Can you work these out from the model? Positions are in its coordinate system, mm. A direction names the side the tool comes from. Coordinates: 2 decimals unless noted, no trailing zeros. Order: outer loops, then holes, each group sorted by start corner. A loop starts at its lowest first (then second) coordinate and runs counter-clockwise, first axis right, second up. Notation, with made-up numbers: (-13, 3.5) - (20, 3.5) arc R17 ccw to (20, 16.5) - close; hole circle Ø10 at (7, 7). An arc over 180 degrees is marked (long way). Use a Markdown table: item, result. Add a question column.
(1) I want a section at C-C (x = -7.5). List the corners of the cut face in (y, z) for me.
(2) We'd pull the mould along Z, two halves only. Please class faces 1 (the cylindrical face through (-35.639, -56.36, -108.857)), 2 (the cylindrical face through (-35.639, -56.36, -32.408)), 3 (the flat face through (0, -24, -10)), 4 (the cylindrical face through (23.66, -15.06, -4.93)): pulls with the +Z half, pulls with the -Z half, needs draft (parallel to the pull), parting line crosses it, or undercut.
(3) I want a section at A-A (z = -64.5). List the corners of the cut face in (x, y) for me, and give its area (3 significant figures).
(4) For pin 1 Ø8 at (y, z) = (-20.5, -3.5) entering from -X; pin 2 Ø11 at (y, z) = (-24.5, -3) entering from +X; pin 3 Ø1 at (x, z) = (0.5, -24.5) entering from +Y, each with a flat end and sliding along its axis, tell me the tip position at first contact or that it passes through.
(5) On a 3-axis mill with a long thin cutter (end or side, diameter ignored), from which of +Z, -Z, +X, -X, +Y, -Y can I reach the whole of each face in a straight line? I mean faces 5 (the flat face through (28.5, -23, -5)), 6 (the flat face through (-17.5, -37, -61)), 7 (the flat face through (17.5, -37, -61)), 8 (the flat face through (-28.5, 23, -5)). Say none if no direction works.
(6) I want a section at D-D (y = -31). List the corners of the cut face in (x, z) for me, and give its area (3 significant figures).
(7) If I drill on L1, parallel to Z at x = -34.5, y = -57; L2, parallel to Y at x = 12.5, z = -80.5; L3, parallel to Z at x = 22, y = 2, over which ranges is the centre line in solid material (lowest first)? Write a range as [from, to].
(8) I want a section at B-B (y = 15). List the corners of the cut face in (x, z) for me, and give its area (3 significant figures).
```python
from build123d import *

# Parameters (mm, degrees)
SKETCH3_W           = 57
SKETCH3_H           = 57
BOSS_EXTRUDE1_DEPTH = 10
SKETCH3_3_R         = 2.55
CUT_EXTRUDE1_DEPTH  = 10
BOSS_EXTRUDE2_DEPTH = 112
SKETCH4_R           = 19.05
SKETCH4_R_2         = 6.5
CUT_EXTRUDE2_DEPTH  = 129.967050055
SKETCH5_R           = 4.15
CUT_EXTRUDE5_DEPTH  = 142.333824685
BOSS_EXTRUDE3_DEPTH = 10
FILLET2_R           = 4
FILLET3_R           = 2
FILLET4_R           = 1


with BuildPart() as part:
    # Sketch3 → Boss-Extrude1 (new body)
    with BuildSketch(Plane.XY):
        Rectangle(SKETCH3_W, SKETCH3_H)
    extrude(amount=-BOSS_EXTRUDE1_DEPTH)

    # Sketch3_3 → Cut-Extrude1 (cut)
    with BuildSketch(Plane.XY):
        with Locations((-24.737446492, 23.520851333)):
            Circle(SKETCH3_3_R)
        with Locations((22.402553508, 23.520851333)):
            Circle(SKETCH3_3_R)
        with Locations(Location((22.402553508, -23.619148667, 0), (0, 0, 180))):
            Circle(SKETCH3_3_R)
        with Locations(Location((-24.737446492, -23.619148667, 0), (0, 0, 180))):
            Circle(SKETCH3_3_R)
        with BuildLine():
            Line((26.210614643, 17.55), (28.5, 17.55))
            Line((28.5, 17.55), (28.5, 12.45))
            Line((28.5, 12.45), (26.210614643, 12.45))
            ThreePointArc((26.210614643, 12.45), (23.660614643, 15), (26.210614643, 17.55))
        make_face()
        with BuildLine():
            Line((26.210614643, -12.45), (28.5, -12.45))
            Line((28.5, -12.45), (28.5, -17.55))
            Line((28.5, -17.55), (26.210614643, -17.55))
            ThreePointArc((26.210614643, -17.55), (23.660614643, -15), (26.210614643, -12.45))
        make_face()
        with BuildLine():
            Line((-26.210614643, -12.45), (-28.5, -12.45))
            Line((-28.5, -12.45), (-28.5, -17.55))
            Line((-28.5, -17.55), (-26.210614643, -17.55))
            ThreePointArc((-26.210614643, -17.55), (-23.660614643, -15), (-26.210614643, -12.45))
        make_face()
        with BuildLine():
            Line((-26.210614643, 17.55), (-28.5, 17.55))
            Line((-28.5, 17.55), (-28.5, 12.45))
            Line((-28.5, 12.45), (-26.210614643, 12.45))
            ThreePointArc((-26.210614643, 12.45), (-23.660614643, 15), (-26.210614643, 17.55))
        make_face()
    extrude(amount=-CUT_EXTRUDE1_DEPTH, mode=Mode.SUBTRACT)

    # Sketch3_4 → Boss-Extrude2 (add)
    with BuildSketch(Plane.XY):
        Polygon((17.5, -46.5), (17.5, -28.5), (-17.5, -28.5), (-17.5, -46.5), (-42.5, -46.5), (-42.5, -66.5), (42.5, -66.5), (42.5, -46.5), align=None)
    extrude(amount=-BOSS_EXTRUDE2_DEPTH)

    # Sketch4 → Cut-Extrude2 (cut, through all)
    # profile 1 of 2: a face of its own
    with BuildSketch(Plane(origin=(0, 0, -10), x_dir=(-1, 0, 0), z_dir=(0, 0, -1))):
        with Locations((-0.070866951, -0.007657079)):
            Circle(SKETCH4_R)
        with Locations((-0.070866951, -0.007657079)):
            Circle(SKETCH4_R_2, mode=Mode.SUBTRACT)
    # profile 2 of 2: a face of its own
    with BuildSketch(Plane(origin=(0, 0, -10), x_dir=(-1, 0, 0), z_dir=(0, 0, -1))):
        with Locations((-0.070866951, -0.007657079)):
            Circle(SKETCH4_R_2)
    extrude(amount=-CUT_EXTRUDE2_DEPTH, mode=Mode.SUBTRACT)

    # Sketch5 → Cut-Extrude5 (cut, through all)
    with BuildSketch(Plane(origin=(0, -46.5, 0), x_dir=(1, 0, 0), z_dir=(0, 1, 0))):
        with Locations(Location((35.955648409, 104.71127815, 0), (0, 0, 270))):
            Circle(SKETCH5_R)
        with Locations(Location((35.955648409, 28.261929333, 0), (0, 0, 270))):
            Circle(SKETCH5_R)
        with Locations(Location((-35.821593513, 28.261929333, 0), (0, 0, 270))):
            Circle(SKETCH5_R)
        with Locations(Location((-35.821593513, 104.71127815, 0), (0, 0, 270))):
            Circle(SKETCH5_R)
    extrude(amount=-CUT_EXTRUDE5_DEPTH, mode=Mode.SUBTRACT)

    # Sketch6 → Boss-Extrude3 (add)
    with BuildSketch(Plane.XY):
        with BuildLine():
            Line((-17.5, -46.5), (-28.5, -28.5))
            ThreePointArc((-28.5, -28.5), (-35.898984404, -36.181212625), (-38.59502311, -46.5))
            Line((-38.59502311, -46.5), (-17.5, -46.5))
        make_face()
        Polygon((-28.5, -28.5), (-17.5, -46.5), (-17.5, -28.5), align=None)
        with BuildLine():
            ThreePointArc((38.59502311, -46.5), (35.898984404, -36.181212625), (28.5, -28.5))
            Line((28.5, -28.5), (17.5, -46.5))
            Line((17.5, -46.5), (38.59502311, -46.5))
        make_face()
        Polygon((17.5, -46.5), (28.5, -28.5), (17.5, -28.5), align=None)
    extrude(amount=-BOSS_EXTRUDE3_DEPTH)

    # Fillet2
    fillet2_edges = [part.edges().sort_by_distance(p)[0] for p in [
        (-38.59502311, -46.5, -5),
        (-28.047511555, -46.5, -10),
    ]]
    fillet(fillet2_edges, radius=FILLET2_R)

    # Fillet3
    fillet3_edges = [part.edges().sort_by_distance(p)[0] for p in [
        (38.59502311, -46.5, -5),
        (28.047511555, -46.5, -10),
    ]]
    fillet(fillet3_edges, radius=FILLET3_R)

    # Fillet4
    fillet4_edges = [part.edges().sort_by_distance(p)[0] for p in [
        (-17.5, -35.5, -10),
        (-17.5, -45.328427125, -11.171572875),
        (17.5, -36.5, -10),
        (17.5, -45.914213562, -10.585786438),
        (0, -28.5, -10),
        (-17.5, -46.5, -63),
        (17.5, -46.5, -62),
    ]]
    fillet(fillet4_edges, radius=FILLET4_R)


solid = part.part
```
Answers follow:
| question | item | result |
|---|---|---|
| 1 | outline | (-66.5, -112) - (-28.5, -112) - (-28.5, -11) arc R1 cw to (-27.5, -10) - (-17.49, -10) - (-17.49, 0) - (-66.5, 0) - close; (17.47, -10) - (28.5, -10) - (28.5, 0) - (17.47, 0) - close |
| 2 | face 1 | undercut |
| 2 | face 2 | undercut |
| 2 | face 3 | pulls with the -Z half |
| 2 | face 4 | needs draft |
| 3 | outline | (-42.5, -66.5) - (42.5, -66.5) - (42.5, -46.5) - (18.5, -46.5) arc R1 cw to (17.5, -45.5) - (17.5, -28.5) - (-17.5, -28.5) - (-17.5, -45.5) arc R1 cw to (-18.5, -46.5) - (-42.5, -46.5) - close |
| 3 | area | 2,330 mm² |
| 4 | pin 1 | stops at x = -28.5 |
| 4 | pin 2 | stops at x = 30.64 |
| 4 | pin 3 | stops at y = -28.5 |
| 5 | face 5 | +Z, -Z, +X, +Y |
| 5 | face 6 | -Z, -X, +Y |
| 5 | face 7 | -Z, +X, +Y |
| 5 | face 8 | +Z, -Z, -X, +Y |
| 6 | outline | (-31.81, -10) - (-18.5, -10) arc R1 cw to (-17.5, -11) - (-17.5, -112) - (17.5, -112) - (17.5, -11) arc R1 cw to (18.5, -10) - (31.81, -10) - (31.81, 0) - (-31.81, 0) - close |
| 6 | area | 4,210 mm² |
| 7 | L1 | z = [-112, -108.65], [-100.78, -32.2], [-24.33, 0] |
| 7 | L2 | y = [-66.5, -28.5] |
| 7 | L3 | z = [-10, 0] |
| 8 | outline | (-23.66, -10) - (-11.66, -10) - (-11.66, 0) - (-23.66, 0) - close; (11.8, -10) - (23.66, -10) - (23.66, 0) - (11.8, 0) - close |
| 8 | area | 239 mm² |
